Work out the finished part from the listing and answer in its coordinate system (mm). Coordinates: 2 decimals unless noted, no trailing zeros. Order: outer loops, then holes, each group sorted by start corner. A loop starts at its lowest first (then second) coordinate and runs counter-clockwise, first axis right, second up. Notation, with made-up numbers: (35.25, 39.5) -> (88.25, 39.5) arc R18 cw to (88.25, 47.5) -> close; hole circle Ø4 at (37, 75). An arc over 180 degrees is marked (long way). Use one line per item in the form item = value.
from build123d import *

# Parameters (mm, degrees)
EXTRUDE_1_DEPTH = 3
FILLET_1_R      = 0.5


with BuildPart() as part:
    # Эскиз1 → Бобышка-Вытянуть1 (new body)
    with BuildSketch(Plane(origin=(0, 0, 0), x_dir=(1, 0, 0), z_dir=(0, 1, 0))):
        Polygon((56.25, 20), (-56.25, 20), (-56.25, 15.425), (-53.25, 15.425), (-53.25, 10.575), (-56.25, 10.575), (-56.25, 7.5), (-62.25, 7.5), (-62.25, -7.5), (-56.25, -7.5), (-56.25, -10.575), (-53.25, -10.575), (-53.25, -15.425), (-56.25, -15.425), (-56.25, -20), (56.25, -20), (56.25, -15.425), (53.25, -15.425), (53.25, -10.575), (56.25, -10.575), (56.25, -7.5), (62.25, -7.5), (62.25, 7.5), (56.25, 7.5), (56.25, 10.575), (53.25, 10.575), (53.25, 15.425), (56.25, 15.425), align=None)
    extrude(amount=EXTRUDE_1_DEPTH)

    # Скругление1
    fillet_1_edges = [part.edges().sort_by_distance(p)[0] for p in [
        (-62.25, 1.5, 7.5),
        (-62.25, 1.5, -7.5),
        (62.25, 1.5, -7.5),
        (62.25, 1.5, 7.5),
    ]]
    fillet(fillet_1_edges, radius=FILLET_1_R)


solid = part.part
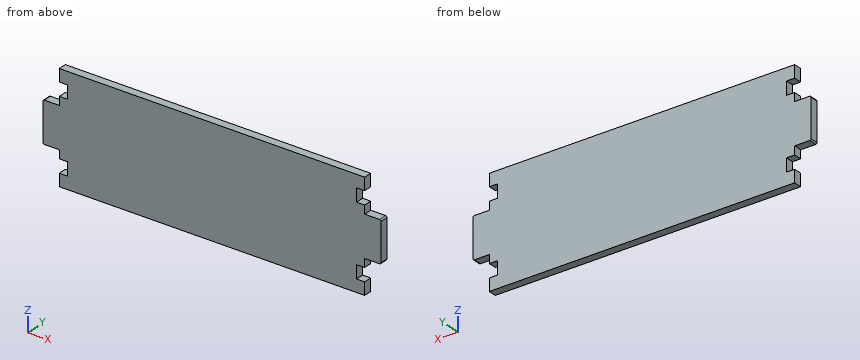
(1) Section B-B on z = 12.5 is taken. Write down the section's boundary in (x, y).
Data:
outline = (-53.25, 0) -> (53.25, 0) -> (53.25, 3) -> (-53.25, 3) -> close
(2) Straight lines are drawn through the part: line 1 along X through (y, z) = (2, 16); line 2 along X through (y, z) = (2.4, -15); line 3 along Z through (x, y) = (56.5, 2.2). For each, find the intervals that lie inside material, in ascending order.
Data:
line_1 = -56.25 to 56.25
line_2 = -53.25 to 53.25
line_3 = -7.5 to 7.5
(3) Each of these flat-tipped pins is pushed along its axis until it touches: P1, Ø1.5, axis at y = 1.5, z = 9, coming from the +X side; P2, Ø0.9, axis at x = -58.5, y = 1, coming from the +Z side; P3, Ø0.9, axis at y = 2, z = -13, coming from the +X side; P4, Ø5, axis at x = 29.5, z = -0.5, coming from the -Y side. Where does it stop, or does it pass through?
Data:
P1 = 56.25
P2 = 7.5
P3 = 53.25
P4 = 0
